Read the model definition and answer for the solid it produces. Units are mm, in the model's axes. A direction names the side the tool comes from. Give positions to 0.01 mm unless a question says otherwise; leave off trailing zeros. Order: outer loops, then holes, each group sorted by start corner. A loop starts at its lowest first (then second) coordinate and runs counter-clockwise, first axis right, second up. Notation, with made-up numbers: M 22,-6 L 68,-6 A33 ccw 68,33 Z; hole C 63,-36.5 d3. An arc over 180 degrees is marked long. One line per item, written item: value. Start each with the question number.
Solid Edge part; units mm, degrees
sketch "Sketch1" plane through (0, 0, 0) normal (0, -1, 0) x (1, 0, 0)
  line L0 (270, 300) -> (100, 0)
  line L1 (100, 0) -> (0, 0)
  line L2 (0, 0) -> (170, 300)
  line L3 (170, 300) -> (270, 300)
extrude "Protrusion1" add sketch "Sketch1" against normal blind 100
sketch "Sketch2" plane through (136.6025, 0, 150) normal (0, -1, 0) x (1, 0, 0)
  line L0 (-108.2692, -100) -> (-108.2692, -150)
  line L1 (-156.6025, -100) -> (-108.2692, -100)
  line L2 (-156.6025, -150) -> (-156.6025, -100)
  line L3 (-136.6025, -150) -> (-156.6025, -150)
extrude "Extrusionsausprägung_2" add sketch "Sketch2" against normal blind 100 material side at (28.3833, 0, 25)
hole "Bohrung_1" at (5, 20, 50) direction (0, 0, -1) diameter 10.5 end up to next start chamfer 1 start chamfer angle 45
hole "Hole1" at (5, 80, 50) direction (0, 0, -1) diameter 10.5 end up to next start chamfer 1 start chamfer angle 45
sketch "Sketch3" plane through (126.0363, 100, 150) normal (0, 1, 0) x (1, 0, 0)
  line L0 (143.9637, -350) -> (143.9637, -150)
  line L1 (143.9637, -150) -> (43.9637, -150)
  line L2 (43.9637, -150) -> (43.9637, -350)
  line L3 (43.9637, -350) -> (143.9637, -350)
extrude "Extrusionsausprägung_3" add sketch "Sketch3" against normal blind 100
hole "Bohrung_5" at (270, 20, 470) direction (-1, 0, 0) diameter 8.376 depth 50 tip angle 118
hole "Hole2" at (270, 80, 470) direction (-1, 0, 0) diameter 8.376 depth 50 tip angle 118
hole "Hole3" at (270, 80, 340) direction (-1, 0, 0) diameter 8.376 depth 50 tip angle 118
hole "Hole4" at (270, 20, 340) direction (-1, 0, 0) diameter 8.376 depth 50 tip angle 118
Q1. Each of these flat-tipped pins is pushed along its axis until it touches: pin 1 (6 mm diameter, centred on y = 74.5, z = 261, fed in from -X); pin 2 (17 mm diameter, centred on x = 5, y = 80, fed in from +Z); pin 3 (10 mm diameter, centred on y = 61.5, z = 437, fed in from -X). Where does it stop, or does it pass through?
Q2. Determine the mould class of faces 1 (the flat face through (169, 100, 230)), 2 (the flat face through (41, 49, 0)), 3 (the cylindrical face through (5.231, 25.245, 24.843)) for opening direction Y: released by +Y, released by -Y, zero draft, split by the parting line, or undercut.
Q3. Find section A-A, the plane x = 5. Give the vertices of the cut face in (y, z), then the cut area to 3 significant figures.
Q4. A tool of negligible diameter and unlimited length cuts with its end or side. For faces 4 (the flat face through (270, 51, 401)), 5 (the flat face through (170, 51, 399)), from which of +Z, -Z, +X, -X, +Y, -Y can it reach the whole face along a straight path? Write none if from no direction.
Q5. Consider probe 1 along Y at (x, z) = (5, 30); probe 2 along Y at (x, z) = (259.5, 340); probe 3 along Z at (x, y) = (258, 80). Determine where each line is inside the solid, lowest interval first.
Q6. Find section D-D, the plane x = 93.5. Give the vertices of the cut face in (y, z).
Q7. Find section B-B, the plane x = 227.5. Give the vertices of the cut face in (y, z), then the cut area to 3 significant figures.
Evaluation:
1. pin 1: x = 146.2
1. pin 2: z = 50
1. pin 3: x = 170
2. face 1: released by +Y
2. face 2: zero draft
2. face 3: undercut
3. outline: M 0,0 L 14.75,0 L 14.75,49 L 13.75,50 L 0,50 Z; M 25.25,0 L 74.75,0 L 74.75,49 L 73.75,50 L 26.25,50 L 25.25,49 Z; M 85.25,0 L 100,0 L 100,50 L 86.25,50 L 85.25,49 Z
3. area: 3,950 mm2
4. face 4: +Z, -Z, +X, +Y, -Y
4. face 5: +Z, -X, +Y, -Y
5. probe 1: 0 to 14.75, 25.25 to 74.75, 85.25 to 100
5. probe 2: 0 to 15.81, 24.19 to 75.81, 84.19 to 100
5. probe 3: 278.82 to 335.81, 344.19 to 465.81, 474.19 to 500
6. outline: M 0,0 L 100,0 L 100,165 L 0,165 Z
7. outline: M 0,225 L 100,225 L 100,500 L 0,500 Z; hole C 20,340 d8.38; hole C 20,470 d8.38; hole C 80,340 d8.38; hole C 80,470 d8.38
7. area: 27,300 mm2
